from build123d import *

# Parameters (mm, degrees)
PAD_DEPTH       = 10
SKETCH005_R     = 1
POCKET001_DEPTH = 10.001
CHAMFER_SIZE    = 9.9


with BuildPart() as part:
    # Sketch → Pad (new body)
    with BuildSketch(Plane.XY):
        with BuildLine():
            ThreePointArc((30.974788, -11.95), (0, 33.2), (-30.974788, -11.95))
            Line((-30.974788, -11.95), (30.974788, -11.95))
        make_face()
    extrude(amount=PAD_DEPTH)

    # Sketch005 (on Face4 of Pad) → Pocket001 (cut, through all)
    with BuildSketch(Plane.XY.offset(10)):
        with Locations((4, -7)):
            Circle(SKETCH005_R)
        with Locations((19.8, -7)):
            Circle(SKETCH005_R)
        with Locations((-4, -7)):
            Circle(SKETCH005_R)
        with Locations((-19.8, -7)):
            Circle(SKETCH005_R)
    extrude(amount=-POCKET001_DEPTH, mode=Mode.SUBTRACT)

    # Chamfer
    chamfer_edges = [part.edges().sort_by_distance(p)[0] for p in [
        (0, 33.2, 0),
    ]]
    chamfer(chamfer_edges, length=CHAMFER_SIZE)


solid = part.part
The model under review builds one solid part; all positions refer to its coordinate system, in mm. Round coordinates to 2 decimals unless told otherwise and drop trailing zeros. Order: outer loops, then holes, each group sorted by start corner. A loop starts at its lowest first (then second) coordinate and runs counter-clockwise, first axis right, second up. Notation, with made-up numbers: (35, 21.25) - (67, 21.25) arc R28 ccw to (67, 60.25) - close; hole circle Ø4 at (-25, 55). An arc over 180 degrees is marked (long way). Use one line per item in the form item = value.
Q1. Add section B-B on y = 0. Give the boundary of the cut face in (x, z).
Response values:
outline = (-33.2, 9.9) - (-23.3, 0) - (23.3, 0) - (33.2, 9.9) - (33.2, 10) - (-33.2, 10) - close
Q2. Clearance check with flat-ended pins moving along their axes: P1, Ø5, axis at y = 19, z = 8.5, coming from the -X side; P2, Ø1.8, axis at x = -19.8, y = -7, coming from the +Z side; P3, Ø5, axis at y = -4.5, z = 8.5, coming from the +X side; P4, Ø3, axis at x = 16.5, z = 7.5, coming from the +Y side. State where each tip first meets the part, or that it passes through.
Response values:
P1 = -28.56
P2 = through
P3 = 33.11
P4 = 27.97
Q3. To check wall thickness, follow line 1 (Y direction, x = -15.5, z = 1); line 2 (Y direction, x = -4, z = 4.25); line 3 (Y direction, x = 0.5, z = 8.75). State the ranges of each line that lie inside material, in increasing order.
Response values:
line_1 = -11.95 to 18.71
line_2 = -11.95 to -8, -6 to 27.26
line_3 = -11.95 to 32.05
Q4. Mouldability with a two-part tool opening along Y and no side actions: class faces 1 (the conical face through (0.7, 23.77, 0.48)), 2 (the flat face through (0, 2, 0)), 3 (the cylindrical face through (-20.8, -7, 5.1)), 4 (the flat face through (0, -11.95, 5)) as pulls with the +Y half, pulls with the -Y half, needs draft (parallel to the pull), parting line crosses it, or undercut.
Response values:
face_1 = parting line crosses it
face_2 = needs draft
face_3 = undercut
face_4 = pulls with the -Y half
Q5. Add section A-A on z = 8.25. Give the boundary of the cut face in (x, y).
Response values:
outline = (-29.2, -11.95) - (29.2, -11.95) arc R31.55 ccw (long way) to start; hole circle Ø2 at (-19.8, -7); hole circle Ø2 at (-4, -7); hole circle Ø2 at (4, -7); hole circle Ø2 at (19.8, -7)
Q6. Add section D-D on z = 1.5. Give the boundary of the cut face in (x, y).
Response values:
outline = (-21.73, -11.95) - (21.73, -11.95) arc R24.8 ccw (long way) to start; hole circle Ø2 at (-19.8, -7); hole circle Ø2 at (-4, -7); hole circle Ø2 at (4, -7); hole circle Ø2 at (19.8, -7)
Q7. Add section C-C on x = 0. Give the boundary of the cut face in (y, z), then the cut area to 3 significant figures.
Response values:
outline = (-11.95, 0) - (23.3, 0) - (33.2, 9.9) - (33.2, 10) - (-11.95, 10) - close
area = 402 mm^2
